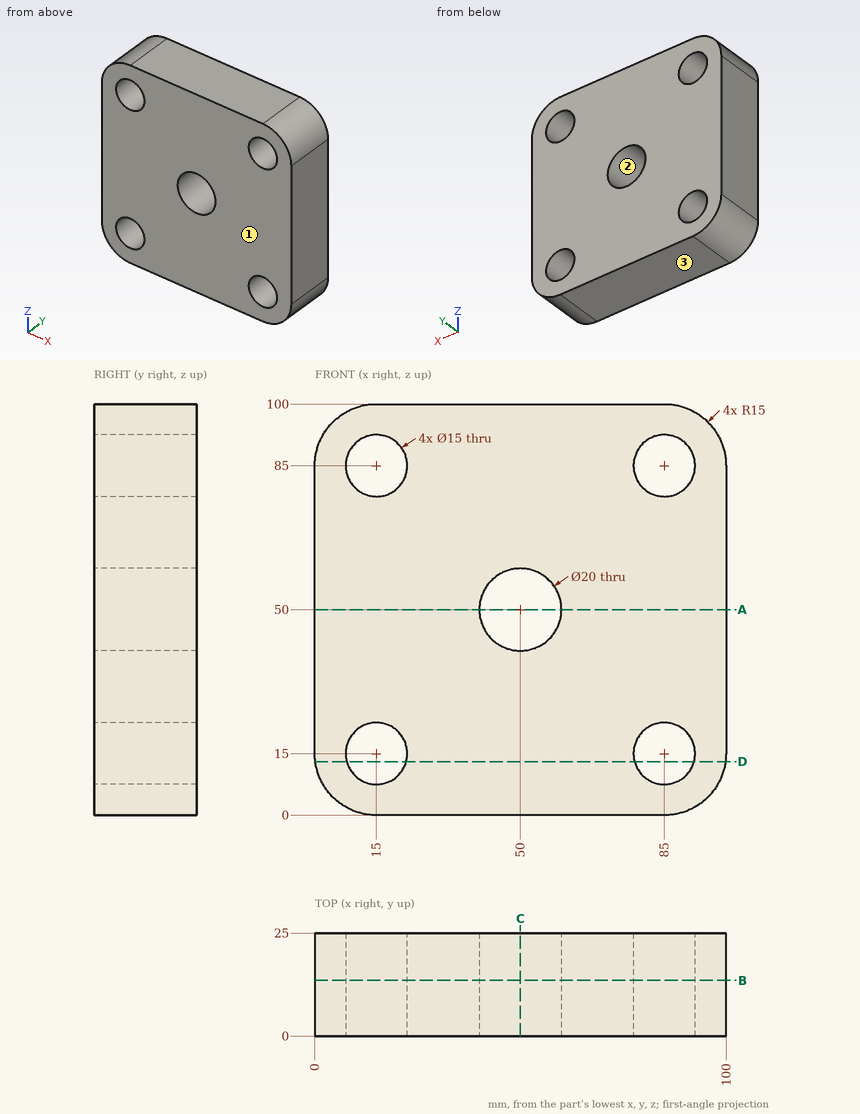
Could you check a few things on this drawing? It's one solid part, dimensions in mm from its lowest x, y, z. Coordinates: 2 decimals unless noted, no trailing zeros. Loops run counter-clockwise (first coordinate to the right, second up) from the corner with the lowest first, then second, coordinate; pieces in that order, holes last. Notation, with made-up numbers: (-40, 54.25) - (-1, 54.25) arc R25 cw to (-1, 71.25) - close; hole circle Ø4 at (13.5, 4). An arc over 180 degrees is marked (long way). Answer as a JSON object with one key per item and string values. Group by question number.
Item 1: If we section it at A-A (z = 50): List the corners of the cut face in (x, y) for me, plus the area to 3 significant figures.
Item 2: If we section it at D-D (z = 13): List the corners of the cut face in (x, y) for me.
Item 3: For pin 1 (24 mm diameter, centred on x = 85, z = 15, fed in from +Y); pin 2 (2 mm diameter, centred on y = 16, z = 89, fed in from +X), each with a flat end and sliding along its axis, tell me the tip position at first contact or that it passes through.
Item 4: If we section it at C-C (x = 50): List the corners of the cut face in (y, z) for me.
Item 5: If we mould it in two halves opening along Z, with no side actions, what happens to the marked faces 1, 2 and 3? For each: released by +Z, released by -Z, zero draft, split by the parting line, or undercut.
Item 6: If we section it at B-B (y = 13.5): List the corners of the cut face in (x, z) for me.
Item 7: If I drill on L1, parallel to Z at x = 85, y = 5.25; L2, parallel to X at y = 1.25, z = 19.5; L3, parallel to X at y = 7.5, z = 88, over which ranges is the centre line in solid material (lowest first)? Write a range as from..to.
Returned:
{
 "1": {"outline": "(0, 0) - (40, 0) - (40, 25) - (0, 25) - close; (60, 0) - (100, 0) - (100, 25) - (60, 25) - close", "area": "2,000 mm²"},
 "2": {"outline": "(0.13, 0) - (7.77, 0) - (7.77, 25) - (0.13, 25) - close; (22.23, 0) - (77.77, 0) - (77.77, 25) - (22.23, 25) - close; (92.23, 0) - (99.87, 0) - (99.87, 25) - (92.23, 25) - close"},
 "3": {"pin 1": "stops at y = 25", "pin 2": "stops at x = 99.7"},
 "4": {"outline": "(0, 0) - (25, 0) - (25, 40) - (0, 40) - close; (0, 60) - (25, 60) - (25, 100) - (0, 100) - close"},
 "5": {"face 1": "zero draft", "face 2": "undercut", "face 3": "released by -Z"},
 "6": {"outline": "(0, 15) arc R15 ccw to (15, 0) - (85, 0) arc R15 ccw to (100, 15) - (100, 85) arc R15 ccw to (85, 100) - (15, 100) arc R15 ccw to (0, 85) - close; hole circle Ø15 at (15, 15); hole circle Ø15 at (15, 85); hole circle Ø20 at (50, 50); hole circle Ø15 at (85, 15); hole circle Ø15 at (85, 85)"},
 "7": {"L1": "z = 0..7.5, 22.5..77.5, 92.5..100", "L2": "x = 0..9, 21..79, 91..100", "L3": "x = 0.3..8.13, 21.87..78.13, 91.87..99.7"}
}
